```python
from build123d import *

# Parameters (mm, degrees)
SKETCH_1_R      = 1.25
SKETCH_1_W      = 8.2
SKETCH_1_H      = 13.2
SKETCH_1_W_2    = 8.4
SKETCH_1_H_2    = 13.4
EXTRUDE_1_DEPTH = 3


with BuildPart() as part:
    # Эскиз1 → Бобышка-Вытянуть1 (new body)
    with BuildSketch(Plane(origin=(0, 0, 0), x_dir=(1, 0, 0), z_dir=(0, 1, 0))):
        with BuildLine():
            Line((-49, 10.671781602), (-49, 67.966339104))
            ThreePointArc((-49, 67.966339104), (-48.707106781, 68.673445885), (-48, 68.966339104))
            Line((-48, 68.966339104), (-27.5, 68.966339104))
            ThreePointArc((-27.5, 68.966339104), (-26.792893219, 69.259232322), (-26.5, 69.966339104))
            Line((-26.5, 69.966339104), (-26.5, 94))
            ThreePointArc((-26.5, 94), (-25.328427125, 96.828427125), (-22.5, 98))
            Line((-22.5, 98), (22.5, 98))
            ThreePointArc((22.5, 98), (25.328427125, 96.828427125), (26.5, 94))
            Line((26.5, 94), (26.5, 69.966339104))
            ThreePointArc((26.5, 69.966339104), (26.792893219, 69.259232322), (27.5, 68.966339104))
            Line((27.5, 68.966339104), (48, 68.966339104))
            ThreePointArc((48, 68.966339104), (48.707106781, 68.673445885), (49, 67.966339104))
            Line((49, 67.966339104), (49, 10.671781602))
            Line((49, 10.671781602), (-49, 10.671781602))
        make_face()
        with Locations(Location((-21.75, 95.624367377, 0), (0, 0, 270))):
            Circle(SKETCH_1_R, mode=Mode.SUBTRACT)
        with Locations(Location((-8.25, 95.624367377, 0), (0, 0, 270))):
            Circle(SKETCH_1_R, mode=Mode.SUBTRACT)
        with Locations(Location((8.25, 95.624367377, 0), (0, 0, 270))):
            Circle(SKETCH_1_R, mode=Mode.SUBTRACT)
        with Locations(Location((21.75, 95.624367377, 0), (0, 0, 270))):
            Circle(SKETCH_1_R, mode=Mode.SUBTRACT)
        with Locations(Location((21.75, 69.808310831, 0), (0, 0, 270))):
            Circle(SKETCH_1_R, mode=Mode.SUBTRACT)
        with Locations(Location((8.25, 69.808310831, 0), (0, 0, 270))):
            Circle(SKETCH_1_R, mode=Mode.SUBTRACT)
        with Locations(Location((-8.25, 69.808310831, 0), (0, 0, 270))):
            Circle(SKETCH_1_R, mode=Mode.SUBTRACT)
        with Locations(Location((-21.75, 69.808310831, 0), (0, 0, 270))):
            Circle(SKETCH_1_R, mode=Mode.SUBTRACT)
        with Locations(Location((-35, 61.966339104, 0), (0, 0, 270))):
            Circle(SKETCH_1_R, mode=Mode.SUBTRACT)
        with Locations(Location((-28, 35.111011166, 0), (0, 0, 270))):
            Circle(SKETCH_1_R, mode=Mode.SUBTRACT)
        with Locations(Location((28, 35.111011166, 0), (0, 0, 270))):
            Circle(SKETCH_1_R, mode=Mode.SUBTRACT)
        with Locations(Location((35, 61.966339104, 0), (0, 0, 270))):
            Circle(SKETCH_1_R, mode=Mode.SUBTRACT)
        with Locations((-43, 19.167635493)):
            Rectangle(SKETCH_1_W, SKETCH_1_H, mode=Mode.SUBTRACT)
        with Locations((43, 19.167635493)):
            Rectangle(SKETCH_1_W, SKETCH_1_H, mode=Mode.SUBTRACT)
        with Locations((0, 89.5)):
            Rectangle(SKETCH_1_W_2, SKETCH_1_H_2, mode=Mode.SUBTRACT)
        Polygon((16, 12.567635493), (-16, 12.567635493), (-18, 14.567635493), (-18, 30.567635493), (-16, 32.567635493), (16, 32.567635493), (18, 30.567635493), (18, 14.567635493), align=None, mode=Mode.SUBTRACT)
    extrude(amount=EXTRUDE_1_DEPTH)


solid = part.part
```
Design review of the part built by this model. Coordinates are the model's own, in mm. A direction names the side the tool comes from. Coordinates: 2 decimals unless noted, no trailing zeros. Loops run counter-clockwise (first coordinate to the right, second up) from the corner with the lowest first, then second, coordinate; pieces in that order, holes last. Notation, with made-up numbers: (-3.75, 77) -> (4.25, 77) arc R17 ccw to (4.25, 88) -> close; hole circle Ø4 at (39, -37.5). An arc over 180 degrees is marked (long way). Answer as a JSON object with one key per item and string values.
Q1. Clearance check with flat-ended pins moving along their axes: pin 1 Ø3 at (x, z) = (-21.75, -95.62) entering from -Y; pin 2 Ø2 at (x, z) = (8.25, -95.62) entering from -Y; pin 3 Ø0.9 at (x, y) = (43.5, 1.5) entering from -Z. State where each tip first meets the part, or that it passes through.
Answer block:
{"pin 1": "stops at y = 0", "pin 2": "passes through", "pin 3": "stops at z = -68.97"}
Q2. To check wall thickness, follow L1, parallel to X at y = 1.7, z = -24; L2, parallel to Z at x = -43, y = 1.55; L3, parallel to X at y = 2.65, z = -28. State the ranges of each line that lie inside material, in increasing order.
Answer block:
{"L1": "x = -49 to -47.1, -38.9 to -18, 18 to 38.9, 47.1 to 49", "L2": "z = -68.97 to -25.77, -12.57 to -10.67", "L3": "x = -49 to -18, 18 to 49"}
Q3. The part is to be moulded in two halves that separate along X. For faces 1 (the flat face through (26.5, 1, -82)), 2 (the flat face through (38, 1, -68.966)), 3 (the cylindrical face through (8.305, 1.479, -71.057)), say which applies: +X half, -X half, draft (parallel to the pull), parting line (faces both ways), or undercut.
Answer block:
{"face 1": "+X half", "face 2": "draft", "face 3": "undercut"}
Q4. Take a section at D-D on z = -62. Give the boundary of the cut face in (x, y), plus the area to 3 significant figures.
Answer block:
{"outline": "(-49, 0) -> (-36.25, 0) -> (-36.25, 3) -> (-49, 3) -> close; (-33.75, 0) -> (33.75, 0) -> (33.75, 3) -> (-33.75, 3) -> close; (36.25, 0) -> (49, 0) -> (49, 3) -> (36.25, 3) -> close", "area": "279 mm^2"}
Q5. Take a section at C-C on x = -8.25. Give the boundary of the cut face in (y, z).
Answer block:
{"outline": "(0, -98) -> (3, -98) -> (3, -96.87) -> (0, -96.87) -> close; (0, -94.37) -> (3, -94.37) -> (3, -71.06) -> (0, -71.06) -> close; (0, -68.56) -> (3, -68.56) -> (3, -32.57) -> (0, -32.57) -> close; (0, -12.57) -> (3, -12.57) -> (3, -10.67) -> (0, -10.67) -> close"}
Q6. Tool access review of faces 4 (the flat face through (17.01, 1.48, -13.58)), 5 (the flat face through (-49, 1, -39)): name each direction out of +Z, -Z, +X, -X, +Y, -Y from which nothing blocks a thin tool from reaching the whole face with its end or side.
Answer block:
{"face 4": "+Y, -Y", "face 5": "+Z, -Z, -X, +Y, -Y"}
Q7. Take a section at B-B on z = -89. Give the boundary of the cut face in (x, y), plus the area to 3 significant figures.
Answer block:
{"outline": "(-26.5, 0) -> (-4.2, 0) -> (-4.2, 3) -> (-26.5, 3) -> close; (4.2, 0) -> (26.5, 0) -> (26.5, 3) -> (4.2, 3) -> close", "area": "134 mm^2"}
Q8. Take a section at A-A on x = 5.5. Give the boundary of the cut face in (y, z), plus the area to 3 significant figures.
Answer block:
{"outline": "(0, -98) -> (3, -98) -> (3, -32.57) -> (0, -32.57) -> close; (0, -12.57) -> (3, -12.57) -> (3, -10.67) -> (0, -10.67) -> close", "area": "202 mm^2"}
